Work out the finished part from the listing and answer in its coordinate system (mm). A direction names the side the tool comes from. Coordinates: 2 decimals unless noted, no trailing zeros. Order: outer loops, then holes, each group sorted by start corner. A loop starts at its lowest first (then second) coordinate and runs counter-clockwise, first axis right, second up. Notation, with made-up numbers: M 17.25,82 L 54.25,82 A5 ccw 54.25,88 Z; hole C 40,-33 d8. An arc over 180 degrees is marked long. Answer in a Markdown table with one row per item. Add a question column.
Item 1: The part is cut by section B-B (z = -22). Write down the section's boundary in (x, y), then the cut area to 3 significant figures.
Item 2: The part is cut by section C-C (y = 20). Write down the section's boundary in (x, z).
Item 3: The part is cut by section D-D (x = 3). Write down the section's boundary in (y, z).
Item 4: Consider line 1 (Y direction, x = 7, z = -31); line 2 (Z direction, x = -6.5, y = 43.5); line 3 (Y direction, x = -19, z = -27). Determine where each line is inside the solid, lowest interval first. Write a range as from..to.
Item 5: Flat-ended cylindrical pins translate along their axes: pin 1 Ø11.5 at (x, y) = (-14.2, -2.5) entering from -Z; pin 2 Ø11 at (x, y) = (-13.95, 20) entering from +Z; pin 3 Ø4 at (x, y) = (-13.95, -25) entering from -Z. Find the tip coordinate at first contact, or state that the pin passes through.
Item 6: The part is cut by section A-A (x = 18.3). Write down the section's boundary in (y, z).
Item 7: The mould has two halves that part along X. Classify faces 1 (the face through (-27, -53, -8.5)), 2 (the face through (0, 52, -15)): released by +X, released by -X, zero draft, split by the parting line, or undercut.
Item 8: Which of the six approach directions +Z, -Z, +X, -X, +Y, -Y give full straight-line access (tool end or side, diameter ignored) to faces 3 (the face through (-14.41, -21.53, 1.01)), 4 (the face through (0, -44, -30)), 5 (the face through (-24.96, 42.06, -31.01)), 6 (the face through (0, -37, -31)), 7 (the face through (24.46, -52.99, -7.56))?
from build123d import *

# Parameters (mm, degrees)
ESBO_O1_W                = 70
ESBO_O1_H                = 108
RESSALTO_EXTRUS_O1_DEPTH = 2
ESBO_O2_W                = 70
ESBO_O2_H                = 2
RESSALTO_EXTRUS_O2_DEPTH = 30
ESBO_O3_W                = 70
ESBO_O3_H                = 17
RESSALTO_EXTRUS_O3_DEPTH = 2
ESBO_O4_R                = 2.5
CORTE_EXTRUS_O1_DEPTH    = 10
ESBO_O8_R                = 2.5
CORTE_EXTRUS_O5_DEPTH    = 10
ESBO_O9_R                = 5
CORTE_EXTRUS_O6_DEPTH    = 10
ESBO_O15_R               = 3.5
CORTE_EXTRUS_O7_DEPTH    = 10
CUT_EXTRUDE1_REACH       = 36
SKETCH1_R                = 2.5


with BuildPart() as part:
    # Esboço1 → Ressalto-extrusão1 (new body)
    with BuildSketch(Plane.XY):
        Rectangle(ESBO_O1_W, ESBO_O1_H)
    extrude(amount=RESSALTO_EXTRUS_O1_DEPTH)

    # Esboço2 → Ressalto-extrusão2 (add)
    with BuildSketch(Plane(origin=(0, 0, 0), x_dir=(-1, 0, 0), z_dir=(0, 0, -1))):
        with Locations((0, -53)):
            Rectangle(ESBO_O2_W, ESBO_O2_H)
    ressalto_extrus_o2 = extrude(amount=RESSALTO_EXTRUS_O2_DEPTH)

    # Esboço3 → Ressalto-extrusão3 (add)
    with BuildSketch(Plane(origin=(0, 0, -30), x_dir=(-1, 0, 0), z_dir=(0, 0, -1))):
        with Locations((0, -45.5)):
            Rectangle(ESBO_O3_W, ESBO_O3_H)
    ressalto_extrus_o3 = extrude(amount=RESSALTO_EXTRUS_O3_DEPTH)

    # Espelhar1: Ressalto-extrusão2, Ressalto-extrusão3 across plane
    add(ressalto_extrus_o2.mirror(Plane.ZX))
    add(ressalto_extrus_o3.mirror(Plane.ZX))

    # Esboço4 → Corte-extrusão1 (cut)
    with BuildSketch(Plane.XY.offset(-30)):
        with Locations((7, -46)):
            Circle(ESBO_O4_R)
        with Locations((18.3, 42.5)):
            Circle(ESBO_O4_R)
    extrude(amount=-CORTE_EXTRUS_O1_DEPTH, mode=Mode.SUBTRACT)

    # Esboço8 → Corte-extrusão5 (cut)
    with BuildSketch(Plane(origin=(0, -52, 0), x_dir=(1, 0, 0), z_dir=(0, 1, 0))):
        with Locations((25, 10)):
            Circle(ESBO_O8_R)
        with Locations((-25, 10)):
            Circle(ESBO_O8_R)
    extrude(amount=-CORTE_EXTRUS_O5_DEPTH, mode=Mode.SUBTRACT)

    # Esboço9 → Corte-extrusão6 (cut)
    with BuildSketch(Plane.XY.offset(2)):
        with Locations((-14.2, -2.5)):
            Circle(ESBO_O9_R)
    extrude(amount=-CORTE_EXTRUS_O6_DEPTH, mode=Mode.SUBTRACT)

    # Esboço15 → Corte-extrusão7 (cut)
    with BuildSketch(Plane.XY.offset(2)):
        with Locations((-13.954549257, 20)):
            Circle(ESBO_O15_R)
        with Locations((-13.954549257, -25)):
            Circle(ESBO_O15_R)
    extrude(amount=-CORTE_EXTRUS_O7_DEPTH, mode=Mode.SUBTRACT)

    # Sketch1 → Cut-Extrude1 (cut, up to next)
    with BuildSketch(Plane(origin=(0, 0, -32), x_dir=(-1, 0, 0), z_dir=(0, 0, -1)), mode=Mode.PRIVATE) as cut_extrude1_sk1:
        with Locations((25.5, 44.5)):
            Circle(SKETCH1_R)
    cut_extrude1_tool1 = extrude(cut_extrude1_sk1.sketch, amount=-CUT_EXTRUDE1_REACH, mode=Mode.PRIVATE) & part.part
    add(cut_extrude1_tool1.solids().sort_by_distance((-25.5, 44.5, -32))[0], mode=Mode.SUBTRACT)
    # Sketch1 → Cut-Extrude1 (cut, up to next)
    with BuildSketch(Plane(origin=(0, 0, -32), x_dir=(-1, 0, 0), z_dir=(0, 0, -1)), mode=Mode.PRIVATE) as cut_extrude1_sk2:
        with Locations((25.5, -44.5)):
            Circle(SKETCH1_R)
    cut_extrude1_tool2 = extrude(cut_extrude1_sk2.sketch, amount=-CUT_EXTRUDE1_REACH, mode=Mode.PRIVATE) & part.part
    add(cut_extrude1_tool2.solids().sort_by_distance((-25.5, -44.5, -32))[0], mode=Mode.SUBTRACT)


solid = part.part
Reply:
| question | item | result |
|---|---|---|
| 1 | outline | M -35,-54 L 35,-54 L 35,-52 L -35,-52 Z; M -35,52 L 35,52 L 35,54 L -35,54 Z |
| 1 | area | 280 mm2 |
| 2 | outline | M -35,0 L -17.45,0 L -17.45,2 L -35,2 Z; M -10.45,0 L 35,0 L 35,2 L -10.45,2 Z |
| 3 | outline | M -54,-32 L -37,-32 L -37,-30 L -52,-30 L -52,0 L 52,0 L 52,-30 L 37,-30 L 37,-32 L 54,-32 L 54,2 L -54,2 Z |
| 4 | line 1 | y = -54..-48.5, -43.5..-37, 37..54 |
| 4 | line 2 | z = -32..-30, 0..2 |
| 4 | line 3 | y = -54..-52, 52..54 |
| 5 | pin 1 | stops at z = 0 |
| 5 | pin 2 | stops at z = 2 |
| 5 | pin 3 | passes through |
| 6 | outline | M -54,-32 L -37,-32 L -37,-30 L -52,-30 L -52,0 L 52,0 L 52,-30 L 45,-30 L 45,-32 L 54,-32 L 54,2 L -54,2 Z; M 37,-32 L 40,-32 L 40,-30 L 37,-30 Z |
| 7 | face 1 | undercut |
| 7 | face 2 | zero draft |
| 8 | face 3 | +Z, -Z |
| 8 | face 4 | +X, -X |
| 8 | face 5 | -Z |
| 8 | face 6 | -Z, +X, -X |
| 8 | face 7 | -Y |
